from build123d import *

# Parameters (mm, degrees)
SKETCH1_W           = 25.4
SKETCH1_H           = 25.4
BOSS_EXTRUDE1_DEPTH = 2.54
SKETCH2_W           = 25.4
SKETCH2_H           = 25.4
BOSS_EXTRUDE2_DEPTH = 2.54
SKETCH3_R           = 3.175
CUT_EXTRUDE1_DEPTH  = 2.54
SKETCH4_R           = 3.175
CUT_EXTRUDE2_DEPTH  = 2.54


with BuildPart() as part:
    # Sketch1 → Boss-Extrude1 (new body)
    with BuildSketch(Plane.XY):
        with Locations((12.7, 12.7)):
            Rectangle(SKETCH1_W, SKETCH1_H)
    extrude(amount=BOSS_EXTRUDE1_DEPTH)

    # Sketch2 → Boss-Extrude2 (add)
    with BuildSketch(Plane(origin=(25.4, 0, 0), x_dir=(0, 0, -1), z_dir=(1, 0, 0))):
        with Locations((-12.7, 12.7)):
            Rectangle(SKETCH2_W, SKETCH2_H)
    extrude(amount=-BOSS_EXTRUDE2_DEPTH)

    # Sketch3 → Cut-Extrude1 (cut)
    with BuildSketch(Plane.XY.offset(2.54)):
        with Locations((11.43, 12.7)):
            Circle(SKETCH3_R)
    extrude(amount=-CUT_EXTRUDE1_DEPTH, mode=Mode.SUBTRACT)

    # Sketch4 → Cut-Extrude2 (cut)
    with BuildSketch(Plane.ZY.offset(-22.86)):
        with Locations((12.7, 12.7)):
            Circle(SKETCH4_R)
    extrude(amount=-CUT_EXTRUDE2_DEPTH, mode=Mode.SUBTRACT)


solid = part.part
Input: part model. Units: mm. Frame: model coordinates. A direction names the side the tool comes from. Give positions to 0.01 mm unless a question says otherwise; leave off trailing zeros. Write each loop counter-clockwise with the first axis right and the second up, starting at its lowest first coordinate (ties: lowest second). Pieces come first, ordered by that corner, then holes. Notation, with made-up numbers: M -17.5,-27.75 L -4.5,-27.75 A26 ccw -4.5,-5.75 Z; hole C -8,54 d1. An arc over 180 degrees is marked long. Use one line per item in the form item = value.
1. Cut plane A-A on z = 12.7. Return loops of the section in (x, y) (3 decimals), and give its area (3 significant figures).
Outcome:
outline = M 22.86,0 L 25.4,0 L 25.4,9.525 L 22.86,9.525 Z; M 22.86,15.875 L 25.4,15.875 L 25.4,25.4 L 22.86,25.4 Z
area = 48.4 mm²
2. First-contact query: P1, Ø3, axis at y = 2.5, z = 16.5, coming from the -X side; P2, Ø1.5, axis at x = 14.5, y = 5, coming from the +Z side. Flat tips, straight axial feed; report the tip coordinate or a pass-through.
Outcome:
P1 = 22.86
P2 = 2.54
3. Cut plane C-C on x = 11.43. Return loops of the section in (y, z) (3 decimals).
Outcome:
outline = M 0,0 L 9.525,0 L 9.525,2.54 L 0,2.54 Z; M 15.875,0 L 25.4,0 L 25.4,2.54 L 15.875,2.54 Z
4. Mould query, pull axis Y, two halves, no side actions, for faces 3 (the face through (24.11, 10.77, 10.18)), 4 (the face through (8.91, 10.77, 1.29)), 5 (the face through (23.1, 25.4, 8.1)), 6 (the face through (14, 10, 2.54)). Classes: released by +Y, released by -Y, zero draft, split by the parting line, or undercut.
Outcome:
face_3 = undercut
face_4 = undercut
face_5 = released by +Y
face_6 = zero draft
5. Ray query, L1, parallel to Y at x = 11.43, z = 0.7 (3 decimals); L2, parallel to Z at x = 10.75, y = 3; L3, parallel to X at y = 8, z = 13.25. Return the intervals inside material, ascending.
Outcome:
L1 = 0 to 9.525, 15.875 to 25.4
L2 = 0 to 2.54
L3 = 22.86 to 25.4
6. Reachability of faces 1 (the face through (22.86, 13, 17)), 2 (the face through (24, 13, 25.4)) from +Z, -Z, +X, -X, +Y, -Y: full face, straight path, thin tool, end or side. Return the list, or none.
Outcome:
face_1 = +Z, -X, +Y, -Y
face_2 = +Z, +X, -X, +Y, -Y
7. Cut plane B-B on y = 12.7. Return loops of the section in (x, z) (3 decimals), and give its area (3 significant figures).
Outcome:
outline = M 0,0 L 8.255,0 L 8.255,2.54 L 0,2.54 Z; M 14.605,0 L 25.4,0 L 25.4,9.525 L 22.86,9.525 L 22.86,2.54 L 14.605,2.54 Z; M 22.86,15.875 L 25.4,15.875 L 25.4,25.4 L 22.86,25.4 Z
area = 90.3 mm²
8. Cut plane D-D on y = 20.5. Return loops of the section in (x, z).
Outcome:
outline = M 0,0 L 25.4,0 L 25.4,25.4 L 22.86,25.4 L 22.86,2.54 L 0,2.54 Z
